Can you work these out from the model? Positions are in its coordinate system, mm. Face numbers are marked on the shaded views. A direction names the side the tool comes from. Round coordinates to 2 decimals unless told otherwise and drop trailing zeros. Write each loop counter-clockwise with the first axis right and the second up, starting at its lowest first coordinate (ties: lowest second). Pieces come first, ordered by that corner, then holes. Notation, with made-up numbers: (47, 72) - (86, 72) arc R19 cw to (86, 76) - close; hole circle Ø6 at (-0.75, -36). An arc over 180 degrees is marked (long way). One line per item, written item: value. Start each with the question number.
(1) I want a section at B-B on z = -4.25. Give the number of separate pieces and of enclosed holes in the cut face, plus the area to 3 significant figures.
(2) On a 3-axis mill with a long thin cutter (end or side, diameter ignored), from which of +Z, -Z, +X, -X, +Y, -Y can I reach the whole of each face in a straight line? I mean the marked faces 4, 5, 6, 7 and 8. Say none if no direction works.
(3) If I drill on L1, parallel to Y at x = 0, z = 0.9; L2, parallel to Y at x = 2.25, z = -1; L3, parallel to Z at x = -1.25, y = 8.5, over which ranges is the centre line in solid material (lowest first)? Write a range as from..to.
(4) I'm going to push flat-ended pins straight in: pin 1 Ø1.5 at (x, y) = (-5, -4) entering from +Z; pin 2 Ø0.6 at (y, z) = (-3.5, -4.5) entering from -X; pin 3 Ø3 at (x, y) = (0, 0) entering from -Z. Where does each tip first touch, or does it pass through?
(5) I want a section at A-A on y = 6.75. List the corners of the cut face in (x, z) for me, plus the area to 3 significant figures.
(6) Thinking about a two-plate mould opening in Y: for the marked faces 1, 2 and 3, which applies, +Y half, -Y half, draft (parallel to the pull), parting line (faces both ways), or undercut?
from build123d import *

# Parameters (mm, degrees)
SKETCH1_R              = 1.27
BOSS_EXTRUDE1_DEPTH    = 1.5875
SKETCH2_W              = 12.7
SKETCH2_H              = 5.0038
SKETCH2_W_2            = 11.176
SKETCH2_H_2            = 3.4798
BOSS_EXTRUDE2_DEPTH    = 5.08
SKETCH4_W              = 5.08
SKETCH4_H              = 6.35
BOSS_EXTRUDE3_DEPTH    = 1.905
SKETCH5_W              = 11.176
SKETCH5_H              = 3.4798
BOSS_EXTRUDE4_DEPTH    = 0.508
SKETCH6_W              = 0.381
SKETCH6_H              = 0.381
BOSS_EXTRUDE5_DEPTH    = 4.064
LPATTERN1_COUNT        = 5
LPATTERN1_PITCH        = 1.5875
SKETCH7_W              = 3.048
SKETCH7_H              = 1.524
BOSS_EXTRUDE6_DEPTH    = 0.8636
SKETCH7_3_W            = 1.524
SKETCH7_3_H            = 0.762
BOSS_EXTRUDE7_DEPTH    = 0.508
SKETCH7_3_W_2          = 1.778
BOSS_EXTRUDE7_2_DEPTH  = 0.508
SKETCH7_4_W            = 0.635
SKETCH7_4_H            = 0.9652
BOSS_EXTRUDE8_DEPTH    = 0.381
BOSS_EXTRUDE8_2_DEPTH  = 0.381
SKETCH7_5_W            = 1.016
SKETCH7_5_H            = 1.778
BOSS_EXTRUDE9_DEPTH    = 1.27
SKETCH7_6_W            = 1.778
SKETCH7_6_H            = 1.016
BOSS_EXTRUDE10_DEPTH   = 0.381
SKETCH7_6_W_2          = 1.016
SKETCH7_6_H_2          = 1.778
BOSS_EXTRUDE10_2_DEPTH = 0.381
SKETCH10_W             = 2.413
SKETCH10_H             = 0.762
CUT_EXTRUDE2_DEPTH     = 2.54


with BuildPart() as part:
    # Sketch1 → Boss-Extrude1 (new body)
    with BuildSketch(Plane.XY):
        with BuildLine():
            Line((-6.35, -9.497254818), (6.35, -9.497254818))
            Line((6.35, -9.497254818), (6.35, 0.580990975))
            ThreePointArc((6.35, 0.580990975), (7.194788478, 1.836453568), (7.794430359, 3.2258))
            Line((7.794430359, 3.2258), (8.0391, 3.2258))
            Line((8.0391, 3.2258), (8.0391, 8.3058))
            Line((8.0391, 8.3058), (7.794430359, 8.3058))
            ThreePointArc((7.794430359, 8.3058), (6.129120563, 11.209936823), (3.4417, 13.206192848))
            Line((3.4417, 13.206192848), (3.4417, 13.819945182))
            Line((3.4417, 13.819945182), (-3.4417, 13.819945182))
            Line((-3.4417, 13.819945182), (-3.4417, 13.206192848))
            ThreePointArc((-3.4417, 13.206192848), (-6.129120563, 11.209936823), (-7.794430359, 8.3058))
            Line((-7.794430359, 8.3058), (-8.0391, 8.3058))
            Line((-8.0391, 8.3058), (-8.0391, 3.2258))
            Line((-8.0391, 3.2258), (-7.794430359, 3.2258))
            ThreePointArc((-7.794430359, 3.2258), (-7.194788478, 1.836453568), (-6.35, 0.580990975))
            Line((-6.35, 0.580990975), (-6.35, -9.497254818))
        make_face()
        Circle(SKETCH1_R, mode=Mode.SUBTRACT)
    extrude(amount=BOSS_EXTRUDE1_DEPTH)


with BuildPart() as body_2:
    # Sketch2 → Boss-Extrude2 (new body)
    with BuildSketch(Plane(origin=(0, 0, 0), x_dir=(-1, 0, 0), z_dir=(0, 0, -1))):
        with Locations((0, -5.547554818)):
            Rectangle(SKETCH2_W, SKETCH2_H)
        with Locations((0, -5.547554818)):
            Rectangle(SKETCH2_W_2, SKETCH2_H_2, mode=Mode.SUBTRACT)
    extrude(amount=BOSS_EXTRUDE2_DEPTH)

    # Sketch10 → Cut-Extrude2 (cut)
    with BuildSketch(Plane(origin=(0, 0, -5.08), x_dir=(-1, 0, 0), z_dir=(0, 0, -1))):
        with Locations((0, -3.426654818)):
            Rectangle(SKETCH10_W, SKETCH10_H)
    extrude(amount=-CUT_EXTRUDE2_DEPTH, mode=Mode.SUBTRACT)


with BuildPart() as body_3:
    # Sketch4 → Boss-Extrude3 (new body)
    with BuildSketch(Plane.XY.offset(1.5875)):
        with Locations((0, 5.7658)):
            Rectangle(SKETCH4_W, SKETCH4_H)
    extrude(amount=BOSS_EXTRUDE3_DEPTH)


with BuildPart() as body_4:
    # Sketch5 → Boss-Extrude4 (new body)
    with BuildSketch(Plane(origin=(0, 0, 0), x_dir=(-1, 0, 0), z_dir=(0, 0, -1))):
        with Locations((0, -5.547554818)):
            Rectangle(SKETCH5_W, SKETCH5_H)
    extrude(amount=BOSS_EXTRUDE4_DEPTH)

    # Sketch6 → Boss-Extrude5 (add)
    with BuildSketch(Plane(origin=(0, 0, -0.508), x_dir=(-1, 0, 0), z_dir=(0, 0, -1))):
        with Locations((3.175, -4.912554818)):
            Rectangle(SKETCH6_W, SKETCH6_H)
        with Locations((3.175, -6.182554818)):
            Rectangle(SKETCH6_W, SKETCH6_H)
    boss_extrude5 = extrude(amount=BOSS_EXTRUDE5_DEPTH)

    # LPattern1: Boss-Extrude5 ×5
    with Locations(*[(i * LPATTERN1_PITCH, 0, 0) for i in range(1, LPATTERN1_COUNT)]):
        add(boss_extrude5)


with BuildPart() as body_5:
    # Sketch7 → Boss-Extrude6 (new body)
    with BuildSketch(Plane(origin=(0, 0, 0), x_dir=(-1, 0, 0), z_dir=(0, 0, -1))):
        with Locations((4.618593555, 3.105353297)):
            Rectangle(SKETCH7_W, SKETCH7_H)
    extrude(amount=BOSS_EXTRUDE6_DEPTH)


with BuildPart() as body_6:
    # Sketch7<3> → Boss-Extrude7 (new body)
    with BuildSketch(Plane(origin=(0, 0, 0), x_dir=(-1, 0, 0), z_dir=(0, 0, -1))):
        with Locations((0, 12.1412)):
            Rectangle(SKETCH7_3_W, SKETCH7_3_H)
    extrude(amount=BOSS_EXTRUDE7_DEPTH)


with BuildPart() as body_7:
    # Sketch7<3> → Boss-Extrude7 2 (new body)
    with BuildSketch(Plane(origin=(0, 0, 0), x_dir=(-1, 0, 0), z_dir=(0, 0, -1))):
        with Locations((4.445, -0.378654818)):
            Rectangle(SKETCH7_3_W_2, SKETCH7_3_H)
    extrude(amount=BOSS_EXTRUDE7_2_DEPTH)


with BuildPart() as body_8:
    # Sketch7<4> → Boss-Extrude8 (new body)
    with BuildSketch(Plane(origin=(0, 0, 0), x_dir=(-1, 0, 0), z_dir=(0, 0, -1))):
        with Locations((-4.700690056, 0.130459395)):
            Rectangle(SKETCH7_4_W, SKETCH7_4_H)
    extrude(amount=BOSS_EXTRUDE8_DEPTH)


with BuildPart() as body_9:
    # Sketch7<4> → Boss-Extrude8 2 (new body)
    with BuildSketch(Plane(origin=(0, 0, 0), x_dir=(-1, 0, 0), z_dir=(0, 0, -1))):
        with Locations((-3.430690056, 0.130459395)):
            Rectangle(SKETCH7_4_W, SKETCH7_4_H)
    extrude(amount=BOSS_EXTRUDE8_2_DEPTH)


with BuildPart() as body_10:
    # Sketch7<5> → Boss-Extrude9 (new body)
    with BuildSketch(Plane(origin=(0, 0, 0), x_dir=(-1, 0, 0), z_dir=(0, 0, -1))):
        with Locations((4.4831, 6.199945182)):
            Rectangle(SKETCH7_5_W, SKETCH7_5_H)
    extrude(amount=BOSS_EXTRUDE9_DEPTH)


with BuildPart() as body_11:
    # Sketch7<6> → Boss-Extrude10 (new body)
    with BuildSketch(Plane(origin=(0, 0, 0), x_dir=(-1, 0, 0), z_dir=(0, 0, -1))):
        with Locations((0.635, 10.7442)):
            Rectangle(SKETCH7_6_W, SKETCH7_6_H)
    extrude(amount=BOSS_EXTRUDE10_DEPTH)


with BuildPart() as body_12:
    # Sketch7<6> → Boss-Extrude10 2 (new body)
    with BuildSketch(Plane(origin=(0, 0, 0), x_dir=(-1, 0, 0), z_dir=(0, 0, -1))):
        with Locations((-4.4831, 7.215945182)):
            Rectangle(SKETCH7_6_W_2, SKETCH7_6_H_2)
    extrude(amount=BOSS_EXTRUDE10_2_DEPTH)


with BuildPart() as part_1:
    add(part.part)

    # Combine2: union body 2, body 11, body 12, body 10, body 9, body 6, body 7, body 5, body 4, body 3, body 8
    add(body_2.part)
    add(body_11.part)
    add(body_12.part)
    add(body_10.part)
    add(body_9.part)
    add(body_6.part)
    add(body_7.part)
    add(body_5.part)
    add(body_4.part)
    add(body_3.part)
    add(body_8.part)


solid = part_1.part
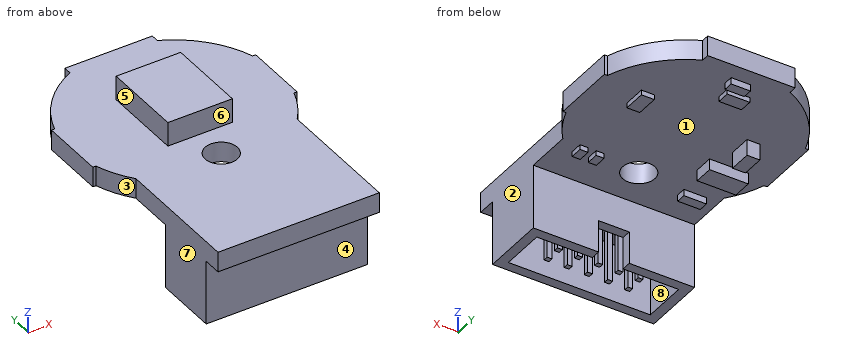
Established:
1. separate pieces: 11
1. enclosed holes: 0
1. area: 24.3 mm2
2. face 4: -Z, +X, -X, -Y
2. face 5: +Z, -X, +Y, -Y
2. face 6: +Z, +X, -X, -Y
2. face 7: +Z, -Z, -X, -Y
2. face 8: -Z
3. L1: -9.5..-1.27, 1.27..13.82
3. L2: -8.05..-7.29, -3.81..-3.05
3. L3: 0..3.49
4. pin 1: z = 1.59
4. pin 2: x = -6.35
4. pin 3: z = 0
5. outline: (-8.04, 0) - (-4.99, 0) - (-4.99, -1.27) - (-3.98, -1.27) - (-3.98, 0) - (3.98, 0) - (3.98, -0.38) - (4.99, -0.38) - (4.99, 0) - (8.04, 0) - (8.04, 1.59) - (2.54, 1.59) - (2.54, 3.49) - (-2.54, 3.49) - (-2.54, 1.59) - (-8.04, 1.59) - close
5. area: 36.9 mm2
6. face 1: undercut
6. face 2: draft
6. face 3: -Y half
